Input: dimensioned drawing with shaded views. Units: mm. Origin: part minimum x, y, z. A direction names the side the tool comes from. Give positions to 0.01 mm unless a question says otherwise; leave off trailing zeros. Write each loop counter-clockwise with the first axis right and the second up, starting at its lowest first coordinate (ties: lowest second). Pieces come first, ordered by that corner, then holes.
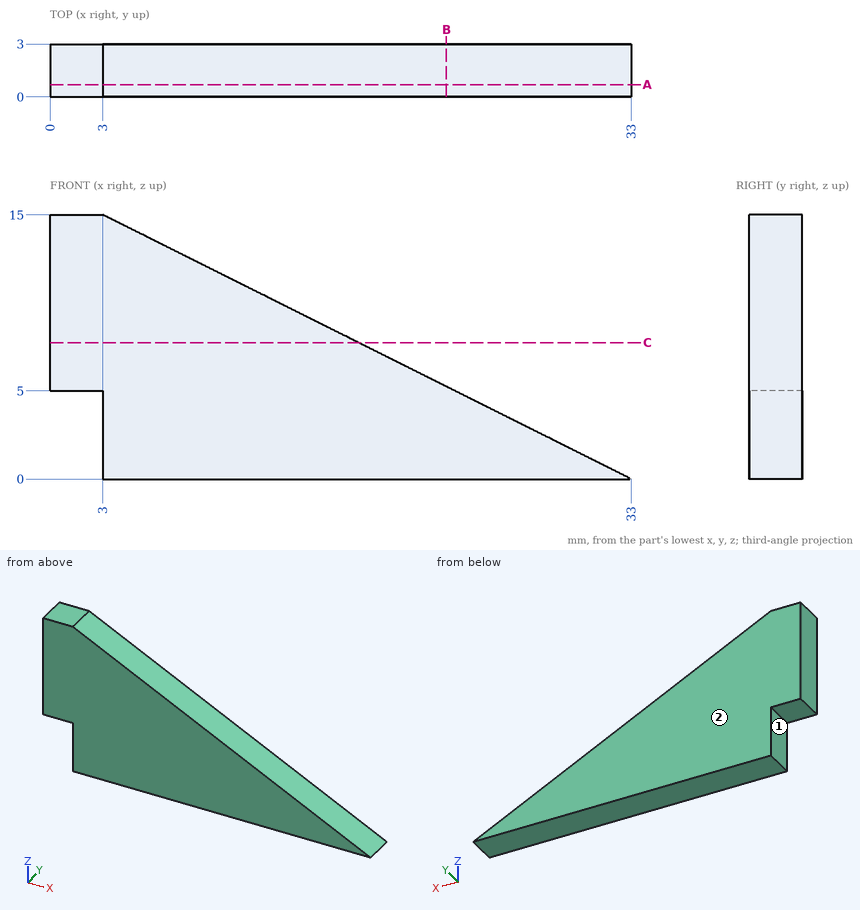
1. Contact query for flat-ended pins moving along their axis: P1, Ø1.5, axis at x = 16.5, y = 1, coming from the +Z side (3 decimals); P2, Ø1.5, axis at y = 2, z = 3, coming from the -X side. Output: stop coordinate, or through.
2. Line query: L1, parallel to Z at x = 27, y = 0.8; L2, parallel to X at y = 1.5, z = 12.5; L3, parallel to X at y = 0.8, z = 12.25. Output: solid intervals per line, ascending.
3. Cut plane B-B, the plane x = 22.5. Return the cut outline in (y, z).
4. Cut plane C-C, the plane z = 7.75. Return the cut outline in (x, y).
5. Access query for the marked faces 1 and 2. Directions: +Z, -Z, +X, -X, +Y, -Y. A direction counts if a zero-diameter tool reaches every point of the face in a straight line with its end or side. Return the directions, or none.
6. Cut plane A-A, the plane y = 0.7. Return the cut outline in (x, z), then the cut area to 3 significant figures.
Response values:
1. P1: stops at z = 8.625
1. P2: stops at x = 3
2. L1: z = 0 to 3
2. L2: x = 0 to 8
2. L3: x = 0 to 8.5
3. outline: (0, 0) - (3, 0) - (3, 5.25) - (0, 5.25) - close
4. outline: (0, 0) - (17.5, 0) - (17.5, 3) - (0, 3) - close
5. face 1: -Z, -X, +Y, -Y
5. face 2: +Z, -Z, +X, -X, +Y
6. outline: (0, 5) - (3, 5) - (3, 0) - (33, 0) - (3, 15) - (0, 15) - close
6. area: 255 mm2
